Can you work these out from the model? Positions are in its coordinate system, mm. A direction names the side the tool comes from. Give positions to 0.01 mm unless a question says otherwise; leave off trailing zeros. Loops run counter-clockwise (first coordinate to the right, second up) from the corner with the lowest first, then second, coordinate; pieces in that order, holes last. Notation, with made-up numbers: (-28, 10.25) -> (29, 10.25) arc R12 cw to (29, 33.25) -> close; hole circle Ø8 at (-19.5, 37.5). An arc over 180 degrees is marked (long way). One line per question, with ' | ' between items.
from build123d import *

# Parameters (mm, degrees)
F0_R     = 14.5
F0_R_2   = 11.5
F1_DEPTH = 13
F2_R     = 14.5
F2_R_2   = 11.5
F3_DEPTH = 3
F4_R     = 3


with BuildPart() as f1:
    # F0 (on Top) → F1 (new body)
    with BuildSketch(Plane.XY):
        Circle(F0_R)
        Circle(F0_R_2, mode=Mode.SUBTRACT)
    extrude(amount=F1_DEPTH)

    # F2 (on face) → F3 (join)
    with BuildSketch(Plane.XY.offset(13)):
        Circle(F2_R)
        Circle(F2_R_2, mode=Mode.SUBTRACT)
        Circle(F2_R_2)
    extrude(amount=F3_DEPTH)

    # F4
    f4_edges = [f1.edges().sort_by_distance(p)[0] for p in [
        (-14.5, 0, 16),
    ]]
    fillet(f4_edges, radius=F4_R)


solid = f1.part
Q1. If we section it at C-C (z = 3.75): Write out the boundary of the cut face in (x, y), plus the area to 3 significant figures.
Entries:
outline: circle Ø29 at (0, 0); hole circle Ø23 at (0, 0) | area: 245 mm²
Q2. If we section it at A-A (y = 0): Write out the boundary of the cut face in (x, z).
Entries:
outline: (-14.5, 0) -> (-11.5, 0) -> (-11.5, 13) -> (11.5, 13) -> (11.5, 0) -> (14.5, 0) -> (14.5, 13) arc R3 ccw to (11.5, 16) -> (-11.5, 16) arc R3 ccw to (-14.5, 13) -> close
Q3. If I drill on probe 1 along Y at (x, z) = (0, 8.5); probe 2 along Z at (x, y) = (-2.75, 1); probe 3 along Y at (x, z) = (-7, 1.5), over which ranges is the centre line in solid material (lowest first)? Write a range as from..to.
Entries:
probe 1: -14.5..-11.5, 11.5..14.5 | probe 2: 13..16 | probe 3: -12.7..-9.12, 9.12..12.7
Q4. If we mould it in two halves opening along Y, with no side actions, what happens to faces 1 (the face through (-9, 8, 0)), 2 (the face through (6.691, -12.864, 6.409)), 3 (the face through (-1.5, 11.4, 6.4))? For each: pulls with the +Y half, pulls with the -Y half, needs draft (parallel to the pull), parting line crosses it, or undercut.
Entries:
face 1: needs draft | face 2: parting line crosses it | face 3: undercut
Q5. For pin 1 Ø8 at (y, z) = (4.5, 5.5) entering from +X; pin 2 Ø1 at (y, z) = (10.5, 12.5) entering from -X; pin 3 Ø8 at (x, z) = (-3, 3) entering from +Y; pin 4 Ø11.5 at (x, y) = (-3.5, -1) entering from -Z, each with a flat end and sliding along its axis, tell me the tip position at first contact or that it passes through.
Entries:
pin 1: x = 14.49 | pin 2: x = -10.5 | pin 3: y = 14.5 | pin 4: z = 13
Q6. On a 3-axis mill with a long thin cutter (end or side, diameter ignored), from which of +Z, -Z, +X, -X, +Y, -Y can I reach the whole of each face in a straight line? I mean faces 4 (the face through (0, 0, 13)), 5 (the face through (0, 0, 16)). Say none if no direction works.
Entries:
face 4: -Z | face 5: +Z, +X, -X, +Y, -Y
